```python
from build123d import *

# Parameters (mm, degrees)
SKETCH1_W           = 98
SKETCH1_H           = 60
BOSS_EXTRUDE1_DEPTH = 1.5
SKETCH2_W           = 98
SKETCH2_H           = 40
BOSS_EXTRUDE2_DEPTH = 9
SKETCH3_W           = 77
SKETCH3_H           = 27
CUT_EXTRUDE1_DEPTH  = 1
SKETCH4_R           = 1.75
CUT_EXTRUDE2_DEPTH  = 2.5
SKETCH5_W           = 42
SKETCH5_H           = 20
BOSS_EXTRUDE3_DEPTH = 9
SKETCH6_W           = 18.449888981
SKETCH6_H           = 44.735350261
SKETCH6_W_2         = 5.736894001
SKETCH6_H_2         = 46.054623325
CUT_EXTRUDE3_DEPTH  = 9


with BuildPart() as part:
    # Sketch1 → Boss-Extrude1 (new body)
    with BuildSketch(Plane.XY):
        Rectangle(SKETCH1_W, SKETCH1_H)
    extrude(amount=BOSS_EXTRUDE1_DEPTH)

    # Sketch2 → Boss-Extrude2 (add)
    with BuildSketch(Plane.XY.offset(1.5)):
        Rectangle(SKETCH2_W, SKETCH2_H)
    extrude(amount=BOSS_EXTRUDE2_DEPTH)

    # Sketch3 → Cut-Extrude1 (cut)
    with BuildSketch(Plane.XY.offset(10.5)):
        Rectangle(SKETCH3_W, SKETCH3_H)
    extrude(amount=-CUT_EXTRUDE1_DEPTH, mode=Mode.SUBTRACT)

    # Sketch4 → Cut-Extrude2 (cut, through all)
    with BuildSketch(Plane.XY.offset(1.5)):
        with Locations((-46.5, 27.5)):
            Circle(SKETCH4_R)
        with Locations((46.5, 27.5)):
            Circle(SKETCH4_R)
        with Locations((46.5, -27.5)):
            Circle(SKETCH4_R)
        with Locations((-46.5, -27.5)):
            Circle(SKETCH4_R)
    extrude(amount=-CUT_EXTRUDE2_DEPTH, mode=Mode.SUBTRACT)

    # Sketch5 → Boss-Extrude3 (add)
    with BuildSketch(Plane(origin=(0, 0, 0), x_dir=(-1, 0, 0), z_dir=(0, 0, -1))):
        with Locations((-19, -18)):
            Rectangle(SKETCH5_W, SKETCH5_H)
    extrude(amount=BOSS_EXTRUDE3_DEPTH)

    # Sketch6 → Cut-Extrude3 (cut)
    with BuildSketch(Plane.XY.offset(10.5)):
        with Locations((-57.724944491, 0.8097006)):
            Rectangle(SKETCH6_W, SKETCH6_H)
        with Locations((51.368447, 0.150064069)):
            Rectangle(SKETCH6_W_2, SKETCH6_H_2)
    extrude(amount=-CUT_EXTRUDE3_DEPTH, mode=Mode.SUBTRACT)


solid = part.part
```
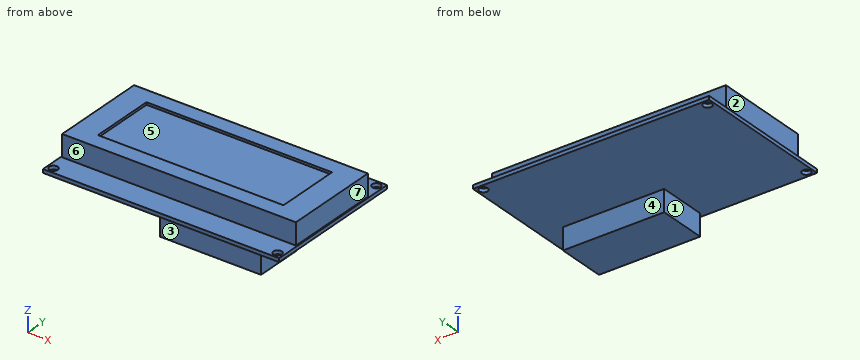
Can you work these out from the model? Positions are in its coordinate system, mm. Face numbers are marked on the shaded views. A direction names the side the tool comes from. Coordinates: 2 decimals unless noted, no trailing zeros. Loops run counter-clockwise (first coordinate to the right, second up) from the corner with the lowest first, then second, coordinate; pieces in that order, holes last.
Item 1: Suppose I cut it at A-A (y = 27.5). Please give me the cut outline in (x, z).
Answers below:
outline: (-49, 0) - (-48.25, 0) - (-48.25, 1.5) - (-49, 1.5) - close; (-44.75, 0) - (44.75, 0) - (44.75, 1.5) - (-44.75, 1.5) - close; (48.25, 0) - (49, 0) - (49, 1.5) - (48.25, 1.5) - close
Item 2: Which directions (+Z, -Z, +X, -X, +Y, -Y) give clear straight access to the entire face, cutting with the end or side of a thin tool? Please do the marked faces 1, 2, 3 and 4.
Answers below:
face 1: -Z, -X, +Y, -Y
face 2: +Z, -X, +Y, -Y
face 3: -Z, +X, -X, -Y
face 4: -Z, +X, -X, +Y
Item 3: I'm going to push flat-ended pins straight in: pin 1 (4.5 mm diameter, centred on x = -46.5, y = -27.5, fed in from +Z); pin 2 (6 mm diameter, centred on x = 12, z = 7, fed in from +Y); pin 3 (7 mm diameter, centred on y = 5.5, z = 5.5, fed in from -X); pin 4 (3 mm diameter, centred on y = 21.5, z = -0.5, fed in from +X). Where does each tip first touch, or does it pass through?
Answers below:
pin 1: stops at z = 1.5
pin 2: stops at y = 20
pin 3: stops at x = -48.5
pin 4: stops at x = 49
Item 4: Suppose I cut it at B-B (x = 46.5). Please give me the cut outline in (y, z).
Answers below:
outline: (-30, 0) - (-29.25, 0) - (-29.25, 1.5) - (-30, 1.5) - close; (-25.75, 0) - (25.75, 0) - (25.75, 1.5) - (20, 1.5) - (20, 10.5) - (-20, 10.5) - (-20, 1.5) - (-25.75, 1.5) - close; (29.25, 0) - (30, 0) - (30, 1.5) - (29.25, 1.5) - close
Item 5: Please list where these lines run through material, in increasing order: L1, parallel to Y at x = -46.5, z = 0.9; L2, parallel to Z at x = -2, y = 8; L3, parallel to Z at x = 19, y = 14.5.
Answers below:
L1: y = -30 to -29.25, -25.75 to 25.75, 29.25 to 30
L2: z = 0 to 9.5
L3: z = 0 to 10.5
Item 6: Suppose I cut it at D-D (z = 2.75). Please give me the cut outline in (x, y), then the cut area to 3 significant figures.
Answers below:
outline: (-48.5, -20) - (48.5, -20) - (48.5, 20) - (-48.5, 20) - close
area: 3,880 mm2
Item 7: Suppose I cut it at C-C (x = -27). Please give me the cut outline in (y, z).
Answers below:
outline: (-30, 0) - (30, 0) - (30, 1.5) - (20, 1.5) - (20, 10.5) - (13.5, 10.5) - (13.5, 9.5) - (-13.5, 9.5) - (-13.5, 10.5) - (-20, 10.5) - (-20, 1.5) - (-30, 1.5) - close
Item 8: If we mould it in two halves opening along Y, with no side actions, what happens to the marked faces 5, 6 and 7? For each: released by +Y, released by -Y, zero draft, split by the parting line, or undercut.
Answers below:
face 5: undercut
face 6: released by -Y
face 7: zero draft
